from build123d import *

# Parameters (mm, degrees)
CROQUIS1_W              = 20
CROQUIS1_H              = 150
CROQUIS1_R              = 4.15
CROQUIS1_W_2            = 5
CROQUIS1_H_2            = 40
CROQUIS1_H_3            = 45
SALIENTE_EXTRUIR1_DEPTH = 4
SALIENTE_EXTRUIR2_START = 4
CROQUIS2_W              = 20
CROQUIS2_H              = 20
CROQUIS2_R              = 4.15
SALIENTE_EXTRUIR2_DEPTH = 30
REDONDEO1_R             = 2
CROQUIS3_R              = 1.875
CORTAR_EXTRUIR1_DEPTH   = 20


with BuildPart() as part:
    # Croquis1 → Saliente-Extruir1 (new body)
    with BuildSketch(Plane.XY):
        with Locations((0, 75)):
            Rectangle(CROQUIS1_W, CROQUIS1_H)
        with Locations((0, 10)):
            Circle(CROQUIS1_R, mode=Mode.SUBTRACT)
        with Locations((0, 125)):
            Rectangle(CROQUIS1_W_2, CROQUIS1_H_2, mode=Mode.SUBTRACT)
        with Locations((0, 70)):
            Rectangle(CROQUIS1_W_2, CROQUIS1_H_3, mode=Mode.SUBTRACT)
    extrude(amount=SALIENTE_EXTRUIR1_DEPTH)

    # Croquis2 → Saliente-Extruir2 (add)
    with BuildSketch(Plane.XY.offset(SALIENTE_EXTRUIR2_START)):
        with Locations((0, 10)):
            Rectangle(CROQUIS2_W, CROQUIS2_H)
        with Locations((0, 10)):
            Circle(CROQUIS2_R, mode=Mode.SUBTRACT)
    extrude(amount=SALIENTE_EXTRUIR2_DEPTH)

    # Redondeo1
    redondeo1_edges = [part.edges().sort_by_distance(p)[0] for p in [
        (-10, 85, 4),
        (10, 85, 4),
        (0, 20, 4),
        (10, 10, 34),
        (0, 20, 34),
        (10, 20, 19),
        (-10, 10, 34),
        (-10, 20, 19),
        (0, 0, 34),
        (10, 0, 17),
        (-10, 0, 17),
    ]]
    fillet(redondeo1_edges, radius=REDONDEO1_R)

    # Croquis3 → Cortar-Extruir1 (cut)
    with BuildSketch(Plane(origin=(0, 0, 0), x_dir=(1, 0, 0), z_dir=(0, 1, 0))):
        with Locations((0, -9)):
            Circle(CROQUIS3_R)
        with Locations((0, -29)):
            Circle(CROQUIS3_R)
        with Locations((0, -19)):
            Circle(CROQUIS3_R)
    extrude(amount=CORTAR_EXTRUIR1_DEPTH, mode=Mode.SUBTRACT)


solid = part.part
Work out the finished part from the listing and answer in its coordinate system (mm). A direction names the side the tool comes from. Round coordinates to 2 decimals unless told otherwise and drop trailing zeros. Order: outer loops, then holes, each group sorted by start corner. A loop starts at its lowest first (then second) coordinate and runs counter-clockwise, first axis right, second up. Notation, with made-up numbers: M 43.5,35 L 94.5,35 A21 ccw 94.5,63 Z; hole C 88,73 d6. An arc over 180 degrees is marked long. One line per item, written item: value.
Q1. Find section C-C on z = 14. Write down the section's boundary in (x, y), then the cut area to 3 significant figures.
Derived:
outline: M -10,2 A2 ccw -8,0 L 8,0 A2 ccw 10,2 L 10,18 A2 ccw 8,20 L -8,20 A2 ccw -10,18 Z; hole C 0,10 d8.3
area: 342 mm²
Q2. Straight lines are drawn through the part: line 1 (Z direction, x = 0, y = 3.5) (3 decimals); line 2 (X direction, y = 16.5, z = 29) (3 decimals); line 3 (Z direction, x = 0, y = 18.5) (1 decimal). For each, find the intervals that lie inside material, in ascending order.
Derived:
line 1: 0 to 7.125, 10.875 to 17.125, 20.875 to 27.125, 30.875 to 34
line 2: -10 to -1.875, 1.875 to 10
line 3: 0 to 7.1, 10.9 to 17.1, 20.9 to 27.1, 30.9 to 33.9
Q3. Find section A-A on z = 29. Write down the section's boundary in (x, y) (3 decimals), then the cut area to 3 significant figures.
Derived:
outline: M -10,2 A2 ccw -8,0 L -1.875,0 L -1.875,6.298 A4.15 cw -1.875,13.702 L -1.875,20 L -8,20 A2 ccw -10,18 Z; M 1.875,0 L 8,0 A2 ccw 10,2 L 10,18 A2 ccw 8,20 L 1.875,20 L 1.875,13.702 A4.15 cw 1.875,6.298 Z
area: 297 mm²
Q4. For faces 1 (the face through (1.73, 3.1, 19.72)), 2 (the face through (-4, 87, 4)), 3 (the face through (2.5, 70, 2)), determine the directions among +Z, -Z, +X, -X, +Y, -Y from which every point of the face is accessible in a straight line to the end or side of a thin tool.
Derived:
face 1: +Y, -Y
face 2: +Z, +X, -X, +Y
face 3: +Z, -Z
Q5. Flat-ended cylindrical pins translate along their axes: pin 1 (5 mm diameter, centred on x = 0.5, z = 14.5, fed in from +Y); pin 2 (2 mm diameter, centred on x = -2.5, y = 105.5, fed in from +Z). Find the tip coordinate at first contact, or state that the pin passes through.
Derived:
pin 1: y = 20
pin 2: z = 4
Q6. Determine the mould class of faces 4 (the face through (4, 76, 0)), 5 (the face through (-2.5, 70, 2)), 6 (the face through (-1.873, 16.807, 18.918)), 7 (the face through (-1.873, 16.807, 28.918)) for opening direction Z: released by +Z, released by -Z, zero draft, split by the parting line, or undercut.
Derived:
face 4: released by -Z
face 5: zero draft
face 6: undercut
face 7: undercut
Q7. Find section B-B on y = 10. Write down the section's boundary in (x, z), then the cut area to 3 significant figures.
Derived:
outline: M -10,0 L -4.15,0 L -4.15,34 L -8,34 A2 ccw -10,32 Z; M 4.15,0 L 10,0 L 10,32 A2 ccw 8,34 L 4.15,34 Z
area: 396 mm²
Q8. Find section D-D on x = 0. Give the number of separate pieces and of enclosed holes in the cut face, then the cut area to 3 significant figures.
Derived:
separate pieces: 10
enclosed holes: 0
area: 445 mm²
